Autodesk Inventor part; units mm, degrees
ref_plane "YZ Plane" through (0, 0, 0) normal (1, 0, 0) x (0, 1, 0)
ref_plane "XZ Plane" through (0, 0, 0) normal (0, 1, 0) x (-1, 0, 0)
ref_plane "XY Plane" through (0, 0, 0) normal (0, 0, 1) x (1, 0, 0)
sketch "스케치1" plane through (0, 0, 0) normal (0, 1, 0) x (-1, 0, 0)
  line L0 (150, 0) -> (150, -250)
  line L1 (150, -250) -> (0, -250) construction
  line L2 (210, 0) -> (-210, 0)
  line L3 (0, -410) -> (0, 360)
  line L4 (100, 0) -> (100, -250) construction
  line L5 (107.4, -198.15) -> (107.4, -201.85)
  line L6 (107.4, -201.85) -> (146.1, -201.85)
  line L7 (146.1, -198.15) -> (107.4, -198.15)
  line L8 (146.1, -201.85) -> (146.1, -198.15)
  line L9 (146.1, 0) -> (146.1, -1.85)
  line L10 (146.1, -1.85) -> (107.4, -1.85)
  line L11 (107.4, -1.85) -> (107.4, 0)
  line L12 (150, 0) -> (150, 250)
  line L13 (150, 250) -> (0, 250)
  line L14 (100, 0) -> (100, 250) construction
  line L15 (146.1, 198.15) -> (107.4, 198.15)
  line L16 (146.1, 201.85) -> (146.1, 198.15)
  line L17 (107.4, 201.85) -> (146.1, 201.85)
  line L18 (107.4, 198.15) -> (107.4, 201.85)
  line L19 (146.1, 0) -> (146.1, 1.85)
  line L20 (146.1, 1.85) -> (107.4, 1.85)
  line L21 (107.4, 1.85) -> (107.4, 0)
  line L22 (-150, 0) -> (-150, -250)
  line L23 (-150, -250) -> (0, -250) construction
  line L24 (-100, 0) -> (-100, -250) construction
  line L25 (-146.1, -198.15) -> (-107.4, -198.15)
  line L26 (-146.1, -201.85) -> (-146.1, -198.15)
  line L27 (-107.4, -201.85) -> (-146.1, -201.85)
  line L28 (-107.4, -198.15) -> (-107.4, -201.85)
  line L29 (-146.1, 0) -> (-146.1, -1.85)
  line L30 (-146.1, -1.85) -> (-107.4, -1.85)
  line L31 (-107.4, -1.85) -> (-107.4, 0)
  line L32 (-146.1, 1.85) -> (-107.4, 1.85)
  line L33 (-146.1, 0) -> (-146.1, 1.85)
  line L34 (-107.4, 1.85) -> (-107.4, 0)
  line L35 (-100, 0) -> (-100, 250) construction
  line L36 (-150, 0) -> (-150, 250)
  line L37 (-146.1, 198.15) -> (-107.4, 198.15)
  line L38 (-107.4, 198.15) -> (-107.4, 201.85)
  line L39 (-146.1, 201.85) -> (-146.1, 198.15)
  line L40 (-107.4, 201.85) -> (-146.1, 201.85)
  line L41 (-150, 250) -> (0, 250)
  line L42 (150, -250) -> (150, -300)
  line L43 (150, -300) -> (-150, -300)
  line L44 (-150, -300) -> (-150, -250)
  line L45 (51.85, -257.4) -> (48.15, -257.4)
  line L46 (48.15, -257.4) -> (48.15, -296.1)
  line L47 (48.15, -296.1) -> (51.85, -296.1)
  line L48 (51.85, -296.1) -> (51.85, -257.4)
  line L49 (-48.15, -257.4) -> (-51.85, -257.4)
  line L50 (-51.85, -257.4) -> (-51.85, -296.1)
  line L51 (-51.85, -296.1) -> (-48.15, -296.1)
  line L52 (-48.15, -296.1) -> (-48.15, -257.4)
  circle A0 centre (0, -150) radius 54
  point P0 (0, 0)
  point P1 (-50, -257.4)
  point P2 (-150, -275)
  point P3 (-51.85, -276.75)
  dimension "d2" = 250
  dimension "d3" = 150
  dimension "d4" = 50
  dimension "d13" = 38.7
  dimension "d14" = 3.7
  dimension "d15" = 48.15
  dimension "d16" = 1.85
  dimension "d17" = 38.7
  dimension "d18" = 7.4
  dimension "d19" = 7.4
  dimension "d20" = 50
  dimension "d21" = 3.7
  dimension "d22" = 38.7
  dimension "d23" = 7.4
  dimension "d24" = 98.15
  dimension "d25" = 38.7
  dimension "d26" = 3.7
  dimension "d27" = 7.4
  dimension "d28" = 98.15
  dimension "d29" = 108
  dimension "d30" = 100
extrude "돌출1" add sketch "스케치1" along normal blind 3.5 contours L0 L42 L43 L3 A0 L2 L11 L10 L9 | L2 L19 L20 L21 L3 L13 L12 | L3 L2 L34 L32 L33 L36 L41 | L43 L44 L22 L2 L29 L30 L31 L3 A0
sketch "스케치5" plane through (0, 3.5, 0) normal (0, 1, 0) x (1, 0, 0)
  point P0 (0, 0)
properties part number "부품1"
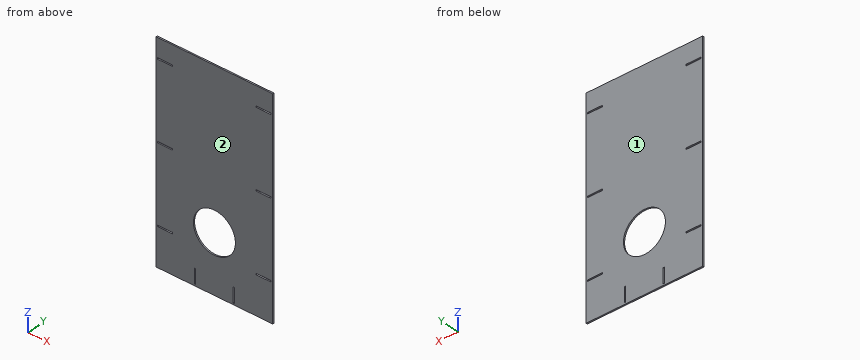
Model file for the job. Use its own axes, mm. Face numbers are marked on the shaded views. Round coordinates to 2 decimals unless told otherwise and drop trailing zeros. Order: outer loops, then holes, each group sorted by start corner. A loop starts at its lowest first (then second) coordinate and runs counter-clockwise, first axis right, second up. Notation, with made-up numbers: M 11,83.5 L 66,83.5 A32 ccw 66,119.5 Z; hole C -34,-7 d1. An arc over 180 degrees is marked long. Write each question's results on one line, items separated by ' | '. Start each with the question number.
(1) Saw through at D-D, the plane y = 2.8. State how many separate pieces and enclosed holes the cut face has, then the cut area to 3 significant figures.
(2) Saw through at B-B, the plane x = 131.5. Give the cut face in (y, z).
(3) Two-plate mould, pull along Y, no slides. Class the marked faces 1 and 2: pulls with the +Y half, pulls with the -Y half, needs draft (parallel to the pull), parting line crosses it, or undercut.
(4) Probe probe 1 along Z at (x, y) = (114, 1.7); probe 2 along Z at (x, y) = (0, 1.7); probe 3 along X at (y, z) = (2.25, -150). List the from-to ranges inside material, lowest first. Write a range as from..to.
(5) Saw through at C-C, the plane x = 0. Give the cut face in (y, z), then the cut area to 3 significant figures.
(6) Saw through at A-A, the plane z = -150. Give the cut face in (x, y).
Established:
1) separate pieces: 1 | enclosed holes: 9 | area: 155,000 mm^2
2) outline: M 0,-300 L 3.5,-300 L 3.5,-201.85 L 0,-201.85 Z; M 0,-198.15 L 3.5,-198.15 L 3.5,-1.85 L 0,-1.85 Z; M 0,1.85 L 3.5,1.85 L 3.5,198.15 L 0,198.15 Z; M 0,201.85 L 3.5,201.85 L 3.5,250 L 0,250 Z
3) face 1: pulls with the +Y half | face 2: pulls with the -Y half
4) probe 1: z = -300..-201.85, -198.15..-1.85, 1.85..198.15, 201.85..250 | probe 2: z = -300..-204, -96..250 | probe 3: x = -150..-54, 54..150
5) outline: M 0,-300 L 3.5,-300 L 3.5,-204 L 0,-204 Z; M 0,-96 L 3.5,-96 L 3.5,250 L 0,250 Z | area: 1,550 mm^2
6) outline: M -150,0 L -54,0 L -54,3.5 L -150,3.5 Z; M 54,0 L 150,0 L 150,3.5 L 54,3.5 Z
